from build123d import *

# Parameters (mm, degrees)
BOSS_EXTRU_1_DEPTH           = 5
ENL_V_MAT_EXTRU_1_REACH      = 322.764
ESQUISSE2_R                  = 2.75
ENL_V_MAT_EXTRU_4_REACH      = 322.764
ESQUISSE6_R                  = 2.25
R_P_TITION_CIRCULAIRE2_COUNT = 3


with BuildPart() as part:
    # Esquisse1 → Boss.-Extru.1 (new body)
    with BuildSketch(Plane(origin=(0, 0, 0), x_dir=(1, 0, 0), z_dir=(0, 1, 0))):
        Polygon((-31.25, 234.548546858), (31.25, 234.548546858), (218.75, -90.210979561), (187.5, -144.337567297), (-187.5, -144.337567297), (-218.75, -90.210979561), align=None)
    extrude(amount=BOSS_EXTRU_1_DEPTH)

    # Esquisse2 → Enl_v. mat.-Extru.1 (cut, up to next)
    with BuildSketch(Plane(origin=(0, 5, 0), x_dir=(1, 0, 0), z_dir=(0, 1, 0)), mode=Mode.PRIVATE) as enl_v_mat_extru_1_sk1:
        with Locations(Location((0, 219.548546858, 0), (0, 0, 270))):
            Circle(ESQUISSE2_R)
    enl_v_mat_extru_1_tool1 = extrude(enl_v_mat_extru_1_sk1.sketch, amount=-ENL_V_MAT_EXTRU_1_REACH, mode=Mode.PRIVATE) & part.part
    # Esquisse2 → Enl_v. mat.-Extru.1 (cut, up to next)
    with BuildSketch(Plane(origin=(0, 5, 0), x_dir=(1, 0, 0), z_dir=(0, 1, 0)), mode=Mode.PRIVATE) as enl_v_mat_extru_1_sk2:
        with Locations(Location((-190.134618943, -109.774273429, 0), (0, 0, 270))):
            Circle(ESQUISSE2_R)
    enl_v_mat_extru_1_tool2 = extrude(enl_v_mat_extru_1_sk2.sketch, amount=-ENL_V_MAT_EXTRU_1_REACH, mode=Mode.PRIVATE) & part.part
    # Esquisse2 → Enl_v. mat.-Extru.1 (cut, up to next)
    with BuildSketch(Plane(origin=(0, 5, 0), x_dir=(1, 0, 0), z_dir=(0, 1, 0)), mode=Mode.PRIVATE) as enl_v_mat_extru_1_sk3:
        with Locations(Location((190.134618943, -109.774273429, 0), (0, 0, 270))):
            Circle(ESQUISSE2_R)
    enl_v_mat_extru_1_tool3 = extrude(enl_v_mat_extru_1_sk3.sketch, amount=-ENL_V_MAT_EXTRU_1_REACH, mode=Mode.PRIVATE) & part.part
    add(enl_v_mat_extru_1_tool1.solids().sort_by_distance((0, 5, -219.548547))[0], mode=Mode.SUBTRACT)
    add(enl_v_mat_extru_1_tool2.solids().sort_by_distance((-190.134619, 5, 109.774273))[0], mode=Mode.SUBTRACT)
    add(enl_v_mat_extru_1_tool3.solids().sort_by_distance((190.134619, 5, 109.774273))[0], mode=Mode.SUBTRACT)

    # Esquisse6 → Enl_v. mat.-Extru.4 (cut, up to next)
    with BuildSketch(Plane(origin=(0, 5, 0), x_dir=(1, 0, 0), z_dir=(0, 1, 0)), mode=Mode.PRIVATE) as enl_v_mat_extru_4_sk1:
        with Locations(Location((-150, -131.337567297, 0), (0, 0, 270))):
            Circle(ESQUISSE6_R)
    enl_v_mat_extru_4_tool1 = extrude(enl_v_mat_extru_4_sk1.sketch, amount=-ENL_V_MAT_EXTRU_4_REACH, mode=Mode.PRIVATE) & part.part
    # Esquisse6 → Enl_v. mat.-Extru.4 (cut, up to next)
    with BuildSketch(Plane(origin=(0, 5, 0), x_dir=(1, 0, 0), z_dir=(0, 1, 0)), mode=Mode.PRIVATE) as enl_v_mat_extru_4_sk2:
        with Locations(Location((150, -131.337567297, 0), (0, 0, 270))):
            Circle(ESQUISSE6_R)
    enl_v_mat_extru_4_tool2 = extrude(enl_v_mat_extru_4_sk2.sketch, amount=-ENL_V_MAT_EXTRU_4_REACH, mode=Mode.PRIVATE) & part.part
    enl_v_mat_extru_4_1 = enl_v_mat_extru_4_tool1.solids().sort_by_distance((-150, 5, 131.337567))[0]
    add(enl_v_mat_extru_4_1, mode=Mode.SUBTRACT)
    enl_v_mat_extru_4_2 = enl_v_mat_extru_4_tool2.solids().sort_by_distance((150, 5, 131.337567))[0]
    add(enl_v_mat_extru_4_2, mode=Mode.SUBTRACT)
    enl_v_mat_extru_4 = enl_v_mat_extru_4_1 + enl_v_mat_extru_4_2  # Enl_v. mat.-Extru.4 as one shape, for the pattern or mirror that repeats it

    # R_p_tition circulaire2: Enl_v. mat.-Extru.4 ×3 about axis
    r_p_tition_circulaire2_axis = Axis((0, 0, 0), (0, 1, 0))
    for i in range(1, R_P_TITION_CIRCULAIRE2_COUNT):
        add(enl_v_mat_extru_4.rotate(r_p_tition_circulaire2_axis, i * 360 / R_P_TITION_CIRCULAIRE2_COUNT), mode=Mode.SUBTRACT)


solid = part.part
CAD build for the part. Positions are in the model's coordinates, mm. Coordinates: 2 decimals unless noted, no trailing zeros. Loops run counter-clockwise (first coordinate to the right, second up) from the corner with the lowest first, then second, coordinate; pieces in that order, holes last. Notation, with made-up numbers: (42.25, 41.25) - (91.25, 41.25) arc R18 cw to (91.25, 59.25) - close; hole circle Ø7 at (-25, -19.5). An arc over 180 degrees is marked (long way). Write item = value, one per line. Start each with the question number.
Q1. Cut at C-C, the plane x = 173. List the corners of the cut face in (y, z), then the cut area to 3 significant figures.
Q2. Drill centre lines: L1, parallel to X at y = 2.25, z = 108.5; L2, parallel to Z at x = -150, y = 1.4; L3, parallel to Z at x = -41.5, y = 1.4. Where is each one in solid material? Low to high.
Q3. Cut at B-B, the plane z = 7. List the corners of the cut face in (x, y).
Q4. Flat gauge pins, fed straight in: pin 1 Ø5 at (x, z) = (188.74, 64.24) entering from -Y; pin 2 Ø1.5 at (y, z) = (0.5, 48) entering from -X. Where does each tip first touch, or does it go through?
Q5. Cut at A-A, the plane y = 3.1. Give the number of separate pieces and of enclosed holes in the cut face, then the cut area to 3 significant figures.
Computed:
q1.outline = (0, 10.97) - (5, 10.97) - (5, 144.34) - (0, 144.34) - close
q1.area = 667 mm²
q2.L1 = -208.19 to -192.57, -187.7 to 187.7, 192.57 to 208.19
q2.L2 = -28.87 to 129.09, 133.59 to 144.34
q2.L3 = -216.8 to 144.34
q3.outline = (-170.71, 0) - (170.71, 0) - (170.71, 5) - (-170.71, 5) - close
q4.pin_1 = 0
q4.pin_2 = -194.81
q5.separate_pieces = 1
q5.enclosed_holes = 9
q5.area = 103,000 mm²
